```python
from build123d import *

# Parameters (mm, degrees)
BOSS_EXTRUDE1_DEPTH = 54
SKETCH2_W           = 3
SKETCH2_H           = 11
CUT_EXTRUDE1_DEPTH  = 20.1
SKETCH3_W           = 19.1
SKETCH3_H           = 36
BOSS_EXTRUDE2_DEPTH = 1.5


with BuildPart() as part:
    # Sketch1 → Boss-Extrude1 (new body)
    with BuildSketch(Plane.XY):
        Polygon((-9.55, 72), (-9.55, 0), (9.55, 0), (9.55, 72), (6.55, 72), (6.55, 32), (6.05, 32), (6.05, 2), (-6.05, 2), (-6.05, 32), (-6.55, 32), (-6.55, 72), align=None)
    extrude(amount=BOSS_EXTRUDE1_DEPTH)

    # Sketch2 → Cut-Extrude1 (cut, through all)
    with BuildSketch(Plane(origin=(9.55, 0, 0), x_dir=(0, 0, -1), z_dir=(1, 0, 0))):
        with Locations((-44.1, 66.5)):
            Rectangle(SKETCH2_W, SKETCH2_H)
        with Locations((-32.7, 66.5)):
            Rectangle(SKETCH2_W, SKETCH2_H)
        with Locations((-21.3, 66.5)):
            Rectangle(SKETCH2_W, SKETCH2_H)
        with Locations((-9.9, 66.5)):
            Rectangle(SKETCH2_W, SKETCH2_H)
    extrude(amount=-CUT_EXTRUDE1_DEPTH, mode=Mode.SUBTRACT)

    # Sketch3 → Boss-Extrude2 (add)
    with BuildSketch(Plane(origin=(0, 0, 0), x_dir=(-1, 0, 0), z_dir=(0, 0, -1))):
        with Locations((0, 18)):
            Rectangle(SKETCH3_W, SKETCH3_H)
    extrude(amount=BOSS_EXTRUDE2_DEPTH)


solid = part.part
```
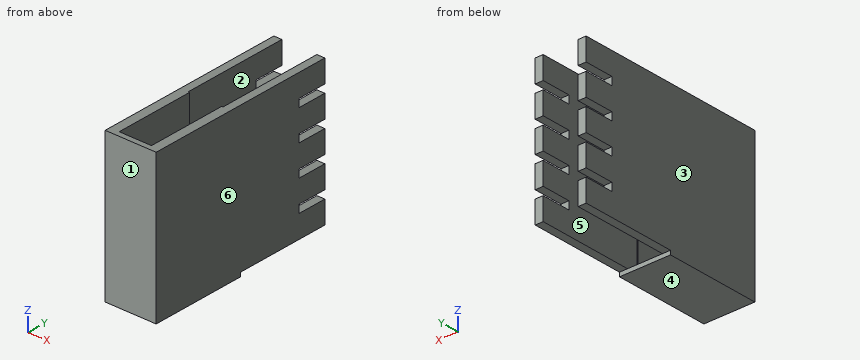
Geometry: final body of the model. Coordinates: model frame, mm. Face numbers are marked on the shaded views. A direction names the side the tool comes from. Round coordinates to 2 decimals unless told otherwise and drop trailing zeros. Order: outer loops, then holes, each group sorted by start corner. A loop starts at its lowest first (then second) coordinate and runs counter-clockwise, first axis right, second up. Notation, with made-up numbers: (28.25, 83) - (37.25, 83) arc R31 cw to (37.25, 121) - close; hole circle Ø8 at (21, -23). An arc over 180 degrees is marked (long way). Use CSV: the item, a comma, the result in double quotes. Start each with the question number.
Q1. Access query for the marked faces 1 and 2. Directions: +Z, -Z, +X, -X, +Y, -Y. A direction counts if a zero-diameter tool reaches every point of the face in a straight line with its end or side. Return the directions, or none.
Q2. Section query C-C (y = 24). Return loops of the section in (x, z), and give its area (3 significant figures).
Q3. Material intervals for line 1 along X through (y, z) = (50, 18.5); line 2 along X through (y, z) = (17.5, 25); line 3 along Y through (x, z) = (6.25, 12.5), sorted ascending. Write a range as from..to.
Q4. Section query A-A (x = 8.25). Return loops of the section in (y, z).
Q5. Section query B-B (y = 37.5). Return loops of the section in (x, z), and give its area (3 significant figures).
Q6. Mould query, pull axis X, two halves, no side actions, for the marked faces 3, 4, 5 and 6. Classes: +X half, -X half, draft (parallel to the pull), parting line (faces both ways), or undercut.
Q7. First-contact query: pin 1 (3.5 mm diameter, centred on x = -8.5, y = 65.5, fed in from -Z); pin 2 (0.9 mm diameter, centred on x = -7.5, z = 44, fed in from +Y); pin 3 (2 mm diameter, centred on x = 5, z = 39, fed in from +Y). Flat tips, straight axial feed; report the tip coordinate or a pass-through.
Q8. Section query D-D (z = 3.5). Return loops of the section in (x, y).
Result set:
1,face 1,"+Z, -Z, +X, -X, -Y"
1,face 2,"+Z, +Y"
2,outline,"(-9.55, -1.5) - (9.55, -1.5) - (9.55, 54) - (6.05, 54) - (6.05, 0) - (-6.05, 0) - (-6.05, 54) - (-9.55, 54) - close"
2,area,"407 mm2"
3,line 1,"x = -9.55..-6.55, 6.55..9.55"
3,line 2,"x = -9.55..-6.05, 6.05..9.55"
3,line 3,"y = 0..32"
4,outline,"(0, -1.5) - (36, -1.5) - (36, 0) - (72, 0) - (72, 8.4) - (61, 8.4) - (61, 11.4) - (72, 11.4) - (72, 19.8) - (61, 19.8) - (61, 22.8) - (72, 22.8) - (72, 31.2) - (61, 31.2) - (61, 34.2) - (72, 34.2) - (72, 42.6) - (61, 42.6) - (61, 45.6) - (72, 45.6) - (72, 54) - (0, 54) - close"
5,outline,"(-9.55, 0) - (-6.55, 0) - (-6.55, 54) - (-9.55, 54) - close; (6.55, 0) - (9.55, 0) - (9.55, 54) - (6.55, 54) - close"
5,area,"324 mm2"
6,face 3,"-X half"
6,face 4,"draft"
6,face 5,"undercut"
6,face 6,"+X half"
7,pin 1,"stops at z = 0"
7,pin 2,"stops at y = 61"
7,pin 3,"stops at y = 2"
8,outline,"(-9.55, 0) - (9.55, 0) - (9.55, 72) - (6.55, 72) - (6.55, 32) - (6.05, 32) - (6.05, 2) - (-6.05, 2) - (-6.05, 32) - (-6.55, 32) - (-6.55, 72) - (-9.55, 72) - close"
